from build123d import *

# Parameters (mm, degrees)
SKETCH1_W           = 55
SKETCH1_H           = 75
SKETCH1_R           = 22.5
BOSS_EXTRUDE1_DEPTH = 7
SKETCH2_R           = 2
CUT_EXTRUDE1_DEPTH  = 15
SKETCH3_R           = 2
CUT_EXTRUDE2_DEPTH  = 15


with BuildPart() as part:
    # Sketch1 → Boss-Extrude1 (new body)
    with BuildSketch(Plane.XY):
        Rectangle(SKETCH1_W, SKETCH1_H)
        Circle(SKETCH1_R, mode=Mode.SUBTRACT)
    extrude(amount=BOSS_EXTRUDE1_DEPTH)

    # Sketch2 → Cut-Extrude1 (cut)
    with BuildSketch(Plane(origin=(0, 37.5, 0), x_dir=(1, 0, 0), z_dir=(0, 1, 0))):
        with Locations((-20, -3.5)):
            Circle(SKETCH2_R)
        with Locations((20, -3.5)):
            Circle(SKETCH2_R)
    extrude(amount=-CUT_EXTRUDE1_DEPTH, mode=Mode.SUBTRACT)

    # Sketch3 → Cut-Extrude2 (cut)
    with BuildSketch(Plane.XZ.offset(37.5)):
        with Locations((-20, 3.5)):
            Circle(SKETCH3_R)
        with Locations((20, 3.5)):
            Circle(SKETCH3_R)
    extrude(amount=-CUT_EXTRUDE2_DEPTH, mode=Mode.SUBTRACT)


solid = part.part
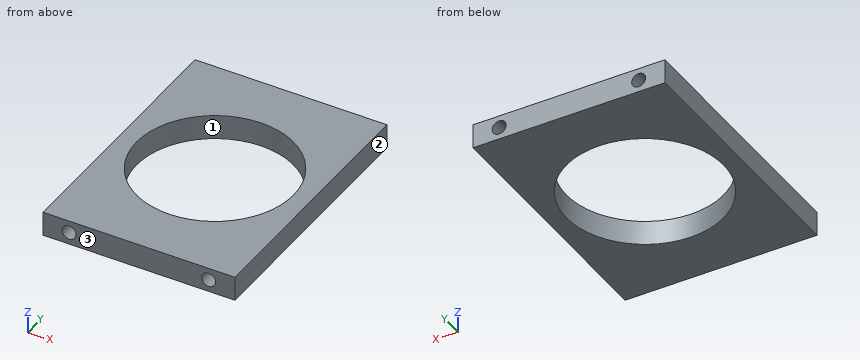
Geometry: final body of the model. Coordinates: model frame, mm. Face numbers are marked on the shaded views. Coordinates: 2 decimals unless noted, no trailing zeros. Order: outer loops, then holes, each group sorted by start corner. A loop starts at its lowest first (then second) coordinate and runs counter-clockwise, first axis right, second up. Notation, with made-up numbers: M 48,-1.75 L 54,-1.75 A10 ccw 54,9.25 Z; hole C 88,-12 d7. An arc over 180 degrees is marked long. One line per question, with ' | ' between items. Start each with the question number.
Item 1: Cut plane C-C, the plane x = 13.5. Return the cut outline in (y, z), then the cut area to 3 significant figures.
Item 2: Cut plane B-B, the plane z = 3.5. Return the cut outline in (x, y).
Item 3: Draft query along X for the marked faces 1, 2 and 3. Return one class per face: released by +X, released by -X, zero draft, split by the parting line, or undercut.
Item 4: Pin query (flat end, axial travel): pin 1 Ø3.5 at (x, z) = (-20, 3.5) entering from -Y; pin 2 Ø1 at (x, y) = (20, 27.5) entering from -Z; pin 3 Ø2 at (x, z) = (19.5, 3) entering from +Y. Return the tip coordinate at first contact, or that it passes through.
Item 5: Cut plane A-A, the plane y = 0. Return the cut outline in (x, z).
Item 6: Cut plane D-D, the plane y = 27.5. Return the cut outline in (x, z), then the cut area to 3 significant figures.
Item 7: Ray query, probe 1 along X at (y, z) = (25.75, 3.5); probe 2 along Z at (x, y) = (-20, 31.5); probe 3 along Y at (x, z) = (0, 3). Return the intervals inside material, ascending. Write a range as [from, to].
A:
1) outline: M -37.5,0 L -18,0 L -18,7 L -37.5,7 Z; M 18,0 L 37.5,0 L 37.5,7 L 18,7 Z | area: 273 mm2
2) outline: M -27.5,-37.5 L -22,-37.5 L -22,-22.5 L -18,-22.5 L -18,-37.5 L 18,-37.5 L 18,-22.5 L 22,-22.5 L 22,-37.5 L 27.5,-37.5 L 27.5,37.5 L 22,37.5 L 22,22.5 L 18,22.5 L 18,37.5 L -18,37.5 L -18,22.5 L -22,22.5 L -22,37.5 L -27.5,37.5 Z; hole C 0,0 d45
3) face 1: undercut | face 2: released by +X | face 3: zero draft
4) pin 1: stops at y = -22.5 | pin 2: stops at z = 0 | pin 3: stops at y = 22.5
5) outline: M -27.5,0 L -22.5,0 L -22.5,7 L -27.5,7 Z; M 22.5,0 L 27.5,0 L 27.5,7 L 22.5,7 Z
6) outline: M -27.5,0 L 27.5,0 L 27.5,7 L -27.5,7 Z; hole C -20,3.5 d4; hole C 20,3.5 d4 | area: 360 mm2
7) probe 1: x = [-27.5, -22], [-18, 18], [22, 27.5] | probe 2: z = [0, 1.5], [5.5, 7] | probe 3: y = [-37.5, -22.5], [22.5, 37.5]
